Answer from the drawing. Dimensions are ordinates in mm from the lowest x, y and z of the part. A direction names the side the tool comes from. Coordinates: 2 decimals unless noted, no trailing zeros. Write each loop counter-clockwise with the first axis right and the second up, starting at its lowest first coordinate (ties: lowest second). Pieces come first, ordered by that corner, then holes.
(1) The mould has two halves that part along Y. Classify the marked faces 1, 2 and 3: +Y half, -Y half, draft (parallel to the pull), parting line (faces both ways), or undercut.
(2) Which of the six approach directions +Z, -Z, +X, -X, +Y, -Y give full straight-line access (tool end or side, diameter ignored) to the marked faces 4 and 5?
(3) Find the intervals of material crossed by probe 1 along Y at (x, z) = (170.5, 3.25); probe 2 along Z at (x, y) = (76.5, 20), in increasing order.
(4) Section A-A on x = 162 is taken. Write down the section's boundary in (y, z).
(5) Section B-B on z = 7.75 is taken. State how many separate pieces and enclosed holes the cut face has, then the cut area to 3 significant figures.
(6) Given pin 1 (12.5 mm diameter, centred on x = 95.5, y = 17, fed in from +Z), flat-ended and moving along its own axis, determine where the tip first touches the part or whether it passes through.
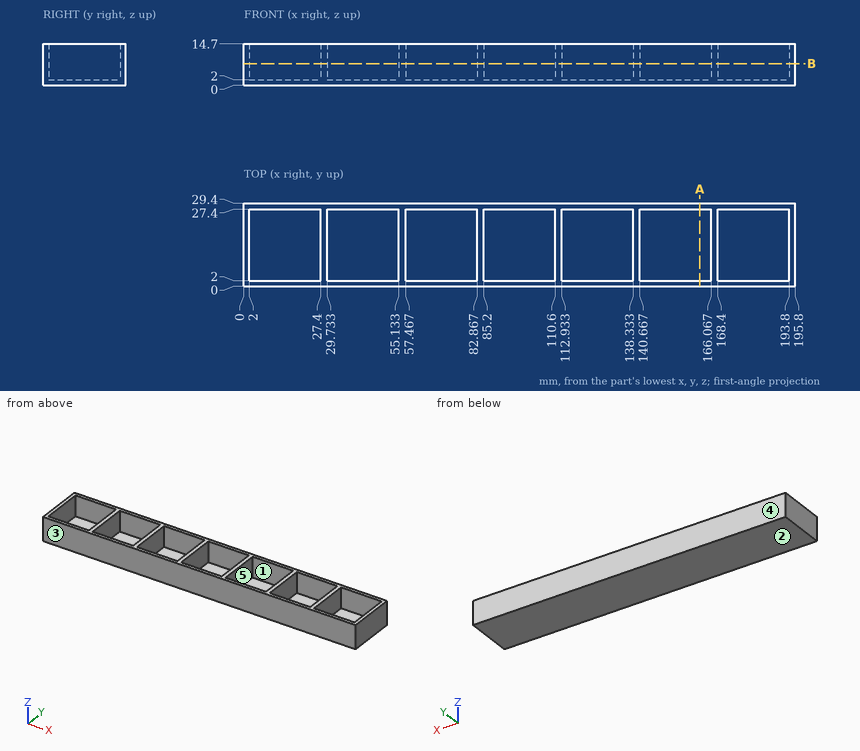
Response:
1. face 1: undercut
1. face 2: draft
1. face 3: -Y half
2. face 4: +Z, -Z, +X, -X, +Y
2. face 5: +Z
3. probe 1: y = 0 to 2, 27.4 to 29.4
3. probe 2: z = 0 to 2
4. outline: (0, 0) - (29.4, 0) - (29.4, 14.7) - (27.4, 14.7) - (27.4, 2) - (2, 2) - (2, 14.7) - (0, 14.7) - close
5. separate pieces: 1
5. enclosed holes: 7
5. area: 1,240 mm2
6. pin 1: stops at z = 2
